from build123d import *

# Parameters (mm, degrees)
SKETCH1_R           = 3.175
SKETCH1_R_2         = 6.35
SKETCH1_R_3         = 0.9
BOSS_EXTRUDE1_DEPTH = 10
FILLET2_R           = 2
FILLET3_R           = 12.7


with BuildPart() as part:
    # Sketch1 → Boss-Extrude1 (new body)
    with BuildSketch(Plane.XY):
        Polygon((-63.5, -12.7), (-63.5, 12.7), (63.5, 12.7), (76.2, 12.7), (76.2, -12.7), (63.5, -12.7), align=None)
        with Locations((-50.8, 0)):
            Circle(SKETCH1_R, mode=Mode.SUBTRACT)
        with Locations((63.5, 0)):
            Circle(SKETCH1_R_2, mode=Mode.SUBTRACT)
        with Locations((63.5, 9.525)):
            Circle(SKETCH1_R_3, mode=Mode.SUBTRACT)
        with Locations((63.5, -9.525)):
            Circle(SKETCH1_R_3, mode=Mode.SUBTRACT)
        with Locations((53.975, 0)):
            Circle(SKETCH1_R_3, mode=Mode.SUBTRACT)
        with Locations((73.025, 0)):
            Circle(SKETCH1_R_3, mode=Mode.SUBTRACT)
        with Locations((-12.7, 0)):
            Circle(SKETCH1_R, mode=Mode.SUBTRACT)
    extrude(amount=BOSS_EXTRUDE1_DEPTH)

    # Fillet2
    fillet2_edges = [part.edges().sort_by_distance(p)[0] for p in [
        (-63.5, -12.7, 5),
        (-63.5, 12.7, 5),
    ]]
    fillet(fillet2_edges, radius=FILLET2_R)

    # Fillet3
    fillet3_edges = [part.edges().sort_by_distance(p)[0] for p in [
        (76.2, 12.7, 5),
        (76.2, -12.7, 5),
    ]]
    fillet(fillet3_edges, radius=FILLET3_R - 0.0001)  # a hair under: the kernel refuses the full size


solid = part.part
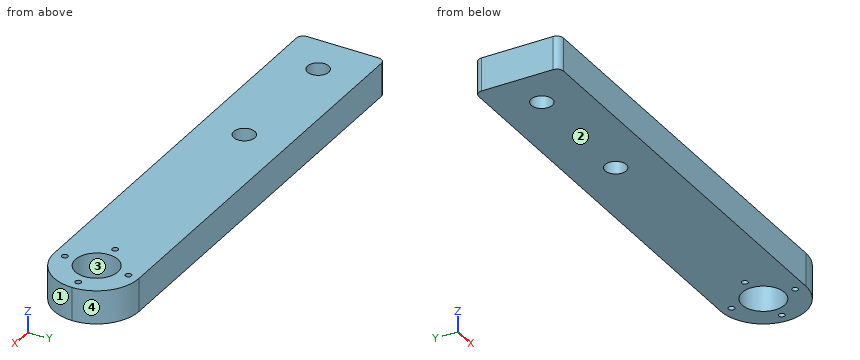
The listing builds one solid part. Answer for the finished solid, in the listing's coordinates (mm). Face numbers are marked on the shaded views. Give positions to 0.01 mm unless a question says otherwise; leave off trailing zeros. Write each loop counter-clockwise with the first axis right and the second up, starting at its lowest first coordinate (ties: lowest second). Pieces come first, ordered by that corner, then holes.
Item 1: Find the intervals of material crossed by line 1 along Y through (x, z) = (63.5, 6.25) (3 decimals); line 2 along Y through (x, z) = (-50.8, 2) (3 decimals); line 3 along X through (y, z) = (5, 7), in increasing order.
Item 2: Section A-A, the plane x = -50.8 is taken. Write down the section's boundary in (y, z) (3 decimals).
Item 3: Section B-B, the plane z = 2 is taken. Count the separate pieces of the cut face and the enclosed holes in it, plus the area to 3 significant figures.
Item 4: Determine the mould class of the marked faces 1, 2, 3 and 4 for opening direction Y: released by +Y, released by -Y, zero draft, split by the parting line, or undercut.
Completed:
1. line 1: y = -12.7 to -10.425, -8.625 to -6.35, 6.35 to 8.625, 10.425 to 12.7
1. line 2: y = -12.7 to -3.175, 3.175 to 12.7
1. line 3: x = -63.5 to 59.59, 67.41 to 75.17
2. outline: (-12.7, 0) - (-3.175, 0) - (-3.175, 10) - (-12.7, 10) - close; (3.175, 0) - (12.7, 0) - (12.7, 10) - (3.175, 10) - close
3. separate pieces: 1
3. enclosed holes: 7
3. area: 3,280 mm2
4. face 1: released by -Y
4. face 2: zero draft
4. face 3: undercut
4. face 4: released by +Y
